Check sheet for the drawn part. Datum: minimum x, y, z corner. Units: mm. A direction names the side the tool comes from. Coordinates: 2 decimals unless noted, no trailing zeros. Order: outer loops, then holes, each group sorted by start corner. A loop starts at its lowest first (then second) coordinate and runs counter-clockwise, first axis right, second up.
Q1. Cross-section at C-C, the plane z = 17. Record the boundary of the cut face in (x, y), and give its area (3 significant figures).
Q2. Thickness scan on line 1 (Z direction, x = 20.5, y = 24); line 2 (X direction, y = 5, z = 3) (1 decimal); line 3 (Z direction, x = 10, y = 18). Record the ranges inside material, lowest first.
Q3. Depth check by flat-ended pin: P1, Ø2, axis at x = 18.5, z = 2, coming from the +Y side; P2, Ø1.2, axis at y = 6.5, z = 1, coming from the -X side (1 decimal); P3, Ø3, axis at y = 4.5, z = 39, coming from the -X side; P4, Ø12.5, axis at x = 27.5, z = 29, coming from the +Y side. Enter the tip coordinate at first touch or a pass-through.
Q4. Cross-section at D-D, the plane y = 13.5. Record the boundary of the cut face in (x, z).
Q5. Set-up check for the marked faces 1, 2 and 3: record each of +Z, -Z, +X, -X, +Y, -Y from which the full face is reachable in a straight line by a thin tool's end or side.
Q6. Cross-section at A-A, the plane y = 6.5. Record the boundary of the cut face in (x, z) (1 decimal).
Q7. Cross-section at B-B, the plane x = 20.5. Record the boundary of the cut face in (y, z), and give its area (3 significant figures).
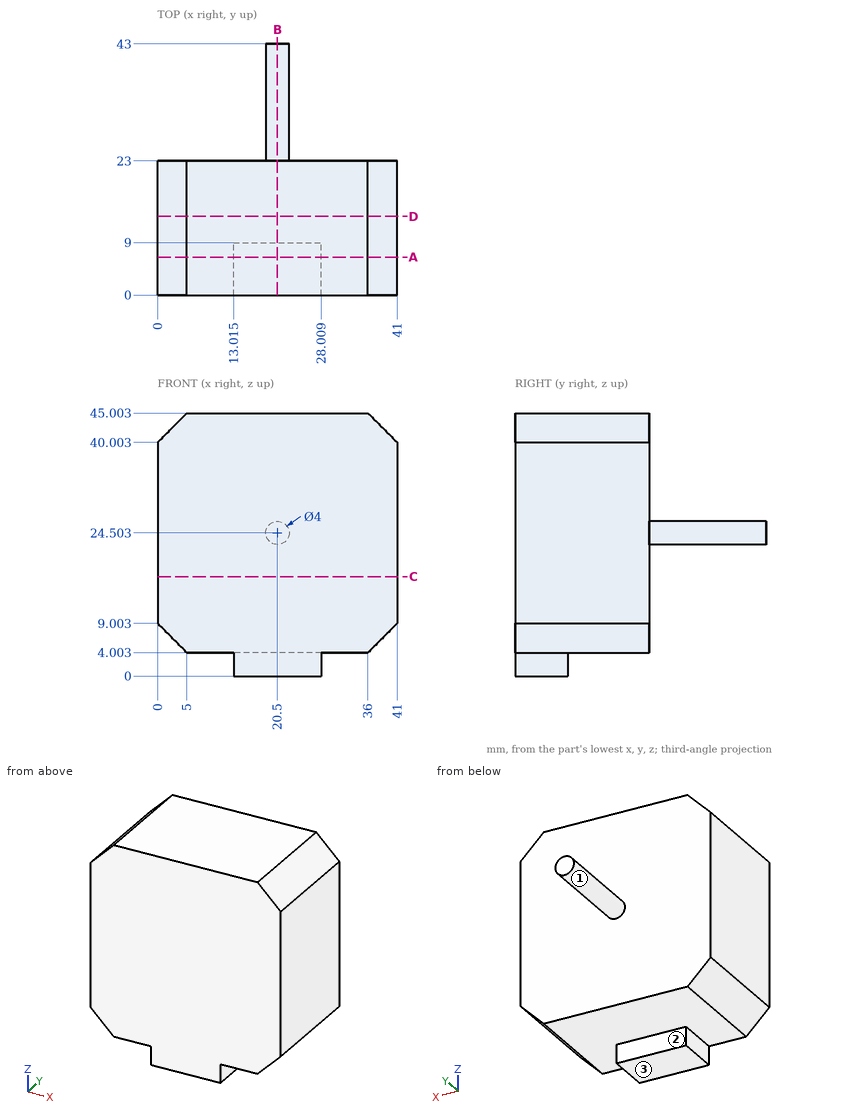
Check values:
1. outline: (0, 0) - (41, 0) - (41, 23) - (0, 23) - close
1. area: 943 mm2
2. line 1: z = 22.5 to 26.5
2. line 2: x = 13 to 28
2. line 3: z = 4 to 45
3. P1: stops at y = 9
3. P2: stops at x = 13
3. P3: stops at x = 0
3. P4: stops at y = 23
4. outline: (0, 9) - (5, 4) - (36, 4) - (41, 9) - (41, 40) - (36, 45) - (5, 45) - (0, 40) - close
5. face 1: +Y
5. face 2: -Z, +X, -X, +Y
5. face 3: -Z, +X, -X, +Y, -Y
6. outline: (0, 9) - (5, 4) - (13, 4) - (13, 0) - (28, 0) - (28, 4) - (36, 4) - (41, 9) - (41, 40) - (36, 45) - (5, 45) - (0, 40) - close
7. outline: (0, 0) - (9, 0) - (9, 4) - (23, 4) - (23, 22.5) - (43, 22.5) - (43, 26.5) - (23, 26.5) - (23, 45) - (0, 45) - close
7. area: 1,060 mm2
